Print and shaded views of the part. All mm, measured from the part's lowest x, y and z. Round coordinates to 2 decimals unless told otherwise and drop trailing zeros. Loops run counter-clockwise (first coordinate to the right, second up) from the corner with the lowest first, then second, coordinate; pieces in that order, holes last. Notation, with made-up numbers: (66, -14) - (110, -14) arc R8 ccw to (110, 1) - close; hole circle Ø1 at (29, 86). An arc over 180 degrees is marked (long way). Use one line per item in the form item = value. Start each with the question number.
Q1. Saw through at A-A (x = 30). Give the cut face in (y, z) (1 decimal), then the cut area to 3 significant figures.
Q2. Drill centre lines: line 1 (Z direction, x = 47.5, y = 3.35); line 2 (Z direction, x = 46, y = 1.05) (1 decimal); line 3 (X direction, y = 1.7, z = 67.5) (1 decimal). Where is each one in solid material? Low to high.
Q3. Saw through at B-B (y = 1.35). Give the cut face in (x, z) (1 decimal).
Q4. Saw through at D-D (x = 88). Give the cut face in (y, z).
Q5. Pin check, flat tips, straight feed: pin 1 (2 mm diameter, centred on y = 1.5, z = 68.5, fed in from +X); pin 2 (6.5 mm diameter, centred on x = 31.15, z = 47.82, fed in from -Y); pin 3 (1 mm diameter, centred on y = 3, z = 45, fed in from -X); pin 4 (3 mm diameter, centred on x = 60.5, y = 3, fed in from +Z) (1 decimal). Stop position of each tip, or through.
Q6. Saw through at C-C (z = 9.5). Give the cut face in (x, y).
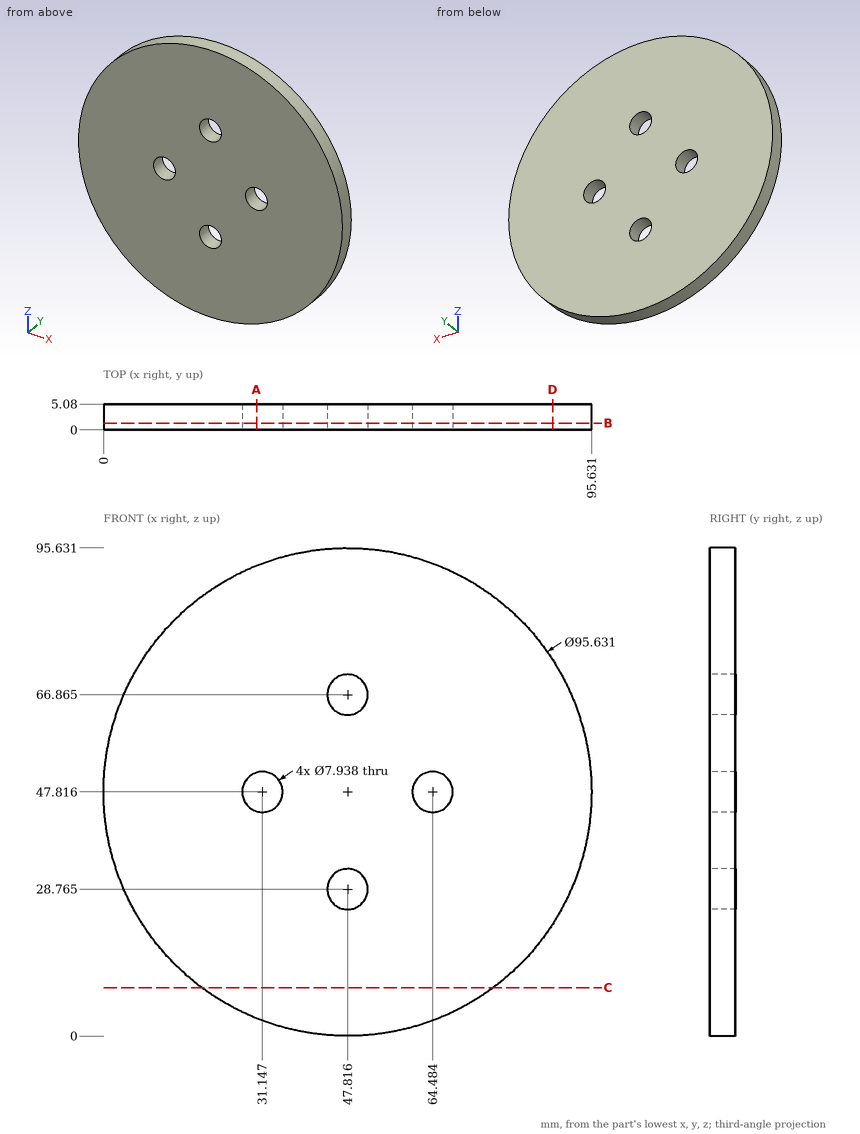
Report:
q1.outline = (0, 3.4) - (5.1, 3.4) - (5.1, 44) - (0, 44) - close; (0, 51.6) - (5.1, 51.6) - (5.1, 92.2) - (0, 92.2) - close
q1.area = 412 mm²
q2.line_1 = 0 to 24.81, 32.72 to 62.91, 70.82 to 95.63
q2.line_2 = 0 to 25.2, 32.3 to 63.3, 70.4 to 95.6
q2.line_3 = 4.2 to 43.9, 51.7 to 91.4
q3.outline = circle Ø95.6 at (47.8, 47.8); hole circle Ø7.9 at (31.1, 47.8); hole circle Ø7.9 at (47.8, 28.8); hole circle Ø7.9 at (47.8, 66.9); hole circle Ø7.9 at (64.5, 47.8)
q4.outline = (0, 21.9) - (5.08, 21.9) - (5.08, 73.73) - (0, 73.73) - close
q5.pin_1 = 91.39
q5.pin_2 = through
q5.pin_3 = 0.06
q5.pin_4 = 94.3
q6.outline = (19.21, 0) - (76.42, 0) - (76.42, 5.08) - (19.21, 5.08) - close
